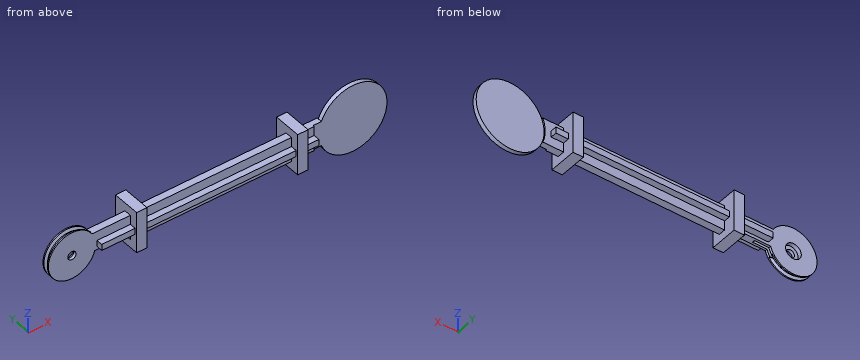
```python
from build123d import *

# Parameters (mm, degrees)
SKETCH1_R                      = 5
BOSS_EXTRUDE1_DEPTH            = 1.7
EP_CABLESLOT_DEPTH             = 0.6
SKETCH4_R                      = 1.9
EP_BALLBEARINGSLOT_DEPTH       = 1
SKETCH5_R                      = 1
EP_SHAFTHOLE_DEPTH             = 0.7
BOSS_EXTRUDE2_START            = -0.85
BOSS_EXTRUDE2_DEPTH            = 1.7
HUMERUSCLEARANCECUT_DEPTH      = 1.7
CABLECLEARANCECUT_DEPTH        = 0.6
SKETCH6_3_R                    = 8.2
MAINPLATE_DEPTH                = 0.5
FINGERPULLEYCLEARANCECUT_DEPTH = 0.35
SKETCH10_W                     = 2.5
SKETCH10_H                     = 10
BLOCK1_DEPTH                   = 3
BLOCK1_DEPTH_BACK              = 3.7
SKETCH13_W                     = 2.5
SKETCH13_H                     = 10
BLOCK2_DEPTH                   = 3
BLOCK2_DEPTH_BACK              = 3.7
SKETCH14_W                     = 36.371319344
SKETCH14_H                     = 1.5
SKETCH14_W_2                   = 5.5
STIFFENERRIB_DEPTH             = 1.5
STIFFENERRIB_DEPTH_BACK        = 3.2


with BuildPart() as part:
    # Sketch1 → Boss-Extrude1 (new body)
    with BuildSketch(Plane(origin=(0, 0, 0), x_dir=(1, 0, 0), z_dir=(0, 1, 0))):
        Circle(SKETCH1_R)
    extrude(amount=BOSS_EXTRUDE1_DEPTH)

    # Sketch2 → Revolve1 (revolve)
    with BuildSketch(Plane.XY):
        Polygon((5, 1.7), (5, 1.15), (5.7, 1.4), (5.7, 1.7), align=None)
        Polygon((5, 0.55), (5, 0), (5.7, 0), (5.7, 0.3), align=None)
    revolve(axis=Axis((0, 1.7, 0), (0, -1, 0)))

    # Sketch3 → EP_CableSlot (cut)
    with BuildSketch(Plane(origin=(0, 0.55, 0), x_dir=(1, 0, 0), z_dir=(0, 1, 0))):
        with BuildLine():
            ThreePointArc((1.166666667, -4.861984049), (2.300738274, -4.439212024), (3.3, -3.756327994))
            Line((3.3, -3.756327994), (3.3, 3.756327994))
            ThreePointArc((3.3, 3.756327994), (2.300738274, 4.439212024), (1.166666667, 4.861984049))
            ThreePointArc((1.166666667, 4.861984049), (2.270562532, 4.155468804), (2.7, 2.917190429))
            Line((2.7, 2.917190429), (2.7, -2.917190429))
            ThreePointArc((2.7, -2.917190429), (2.270562532, -4.155468804), (1.166666667, -4.861984049))
        make_face()
    extrude(amount=EP_CABLESLOT_DEPTH, mode=Mode.SUBTRACT)

    # Sketch4 → EP_BallBearingSlot (cut)
    with BuildSketch(Plane(origin=(0, 1.7, 0), x_dir=(1, 0, 0), z_dir=(0, 1, 0))):
        Circle(SKETCH4_R)
    extrude(amount=-EP_BALLBEARINGSLOT_DEPTH, mode=Mode.SUBTRACT)

    # Sketch5 → EP_ShaftHole (cut)
    with BuildSketch(Plane(origin=(0, 0.7, 0), x_dir=(1, 0, 0), z_dir=(0, 1, 0))):
        Circle(SKETCH5_R)
    extrude(amount=-EP_SHAFTHOLE_DEPTH, mode=Mode.SUBTRACT)

    # Sketch6 → Boss-Extrude2 (add)
    with BuildSketch(Plane(origin=(0, 0.85, 0), x_dir=(1, 0, 0), z_dir=(0, 1, 0)).offset(BOSS_EXTRUDE2_START)):
        with BuildLine():
            ThreePointArc((4, 3), (5, 0), (4, -3))
            Line((4, -3), (60.468486389, -3))
            ThreePointArc((60.468486389, -3), (59.9, 0), (60.468486389, 3))
            Line((60.468486389, 3), (4, 3))
        make_face()
    extrude(amount=BOSS_EXTRUDE2_DEPTH)

    # Sketch8 → HumerusClearanceCut (cut)
    with BuildSketch(Plane(origin=(0, 1.7, 0), x_dir=(1, 0, 0), z_dir=(0, 1, 0))):
        with BuildLine():
            ThreePointArc((4.846648326, 3), (5.22695702, 2.273525963), (5.499090834, 1.5))
            Line((5.499090834, 1.5), (11.499090834, 1.5))
            ThreePointArc((11.499090834, 1.5), (12.999090834, 1.901923789), (14.097167045, 3))
            Line((14.097167045, 3), (4.846648326, 3))
        make_face()
    extrude(amount=-HUMERUSCLEARANCECUT_DEPTH, mode=Mode.SUBTRACT)

    # Sketch11 → CableClearanceCut (cut)
    with BuildSketch(Plane(origin=(0, 0.55, 0), x_dir=(1, 0, 0), z_dir=(0, 1, 0))):
        with BuildLine():
            Line((8.999090834, 1.5), (5.499090834, 1.5))
            ThreePointArc((5.499090834, 1.5), (5.641017612, -0.817875483), (4.846648326, -3))
            ThreePointArc((4.846648326, -3), (4.563342119, -3.415539299), (4.2445102, -3.804488555))
            Line((4.2445102, -3.804488555), (8.999090834, 1.5))
        make_face()
        with BuildLine():
            ThreePointArc((4.846648326, -3), (5.641017612, -0.817875483), (5.499090834, 1.5))
            ThreePointArc((5.499090834, 1.5), (5.22695702, 2.273525963), (4.846648326, 3))
            Line((4.846648326, 3), (4, 3))
            ThreePointArc((4, 3), (5, 0), (4, -3))
            Line((4, -3), (4.846648326, -3))
        make_face()
    extrude(amount=CABLECLEARANCECUT_DEPTH, mode=Mode.SUBTRACT)

    # Sketch6<3> → MainPlate (add, symmetric)
    with BuildSketch(Plane(origin=(0, 0.85, 0), x_dir=(1, 0, 0), z_dir=(0, 1, 0))):
        with Locations((68.1, 0)):
            Circle(SKETCH6_3_R)
    extrude(amount=MAINPLATE_DEPTH, both=True)

    # Sketch12 → FingerPulleyClearanceCut (cut)
    with BuildSketch(Plane(origin=(0, 0, 0), x_dir=(1, 0, 0), z_dir=(0, 1, 0))):
        with BuildLine():
            ThreePointArc((60.468486389, -3), (59.9, 0), (60.468486389, 3))
            Line((60.468486389, 3), (58.468486389, 3))
            Line((58.468486389, 3), (58.468486389, -3))
            Line((58.468486389, -3), (60.468486389, -3))
        make_face()
    extrude(amount=FINGERPULLEYCLEARANCECUT_DEPTH, mode=Mode.SUBTRACT)

    # Sketch10 → Block1 (add, two sides)
    with BuildSketch(Plane(origin=(0, 1.7, 0), x_dir=(1, 0, 0), z_dir=(0, 1, 0))) as block1_sk:
        with Locations((15.347167045, 0)):
            Rectangle(SKETCH10_W, SKETCH10_H)
    extrude(amount=BLOCK1_DEPTH)
    extrude(block1_sk.sketch, amount=-BLOCK1_DEPTH_BACK)

    # Sketch13 → Block2 (add, two sides)
    with BuildSketch(Plane(origin=(0, 1.7, 0), x_dir=(1, 0, 0), z_dir=(0, 1, 0))) as block2_sk:
        with Locations((54.218486389, 0)):
            Rectangle(SKETCH13_W, SKETCH13_H)
    extrude(amount=BLOCK2_DEPTH)
    extrude(block2_sk.sketch, amount=-BLOCK2_DEPTH_BACK)

    # Sketch14 → StiffenerRib (add, two sides)
    with BuildSketch(Plane(origin=(0, 1.7, 0), x_dir=(1, 0, 0), z_dir=(0, 1, 0))) as stiffenerrib_sk:
        with BuildLine():
            Line((16.597167045, -0.75), (16.597167045, 0.75))
            Line((16.597167045, 0.75), (6.053717866, 0.75))
            ThreePointArc((6.053717866, 0.75), (6.1, 0), (6.053717866, -0.75))
            Line((6.053717866, -0.75), (16.597167045, -0.75))
        make_face()
        with Locations((34.782826717, 0)):
            Rectangle(SKETCH14_W, SKETCH14_H)
        with Locations((55.718486389, 0)):
            Rectangle(SKETCH14_W_2, SKETCH14_H)
    extrude(amount=STIFFENERRIB_DEPTH)
    extrude(stiffenerrib_sk.sketch, amount=-STIFFENERRIB_DEPTH_BACK)


solid = part.part
```
CAD build for the part. Positions are in the model's coordinates, mm. Give positions to 0.01 mm unless a question says otherwise; leave off trailing zeros. Write each loop counter-clockwise with the first axis right and the second up, starting at its lowest first coordinate (ties: lowest second). Pieces come first, ordered by that corner, then holes. Notation, with made-up numbers: M -14.75,-14.5 L -2.75,-14.5 A32 ccw -2.75,18.5 Z; hole C -8.75,-21.75 d2. An arc over 180 degrees is marked long. Return JSON: item names as keys, results as strings. Group by question number.
(1) Band-saw the part on D-D (x = 68.1). Give the cut face in (y, z).
(2) Band-saw the part on B-B (x = 25). Give the cut face in (y, z), and give its area (3 significant figures).
(3) Band-saw the part on C-C (z = 0). State how many separate pieces and enclosed holes the cut face has, and give its area (3 significant figures).
(4) Band-saw the part on A-A (x = 0). Give the cut face in (y, z).
(5) Flat gauge pins, fed straight in: pin 1 Ø1.5 at (x, z) = (5.5, -0.5) entering from -Y; pin 2 Ø1.2 at (x, y) = (38, 2.5) entering from +Z; pin 3 Ø1.2 at (x, y) = (9.5, -1) entering from -Z. Where does each tip first touch, or does it go through?
(6) Drill centre lines: L1, parallel to X at y = 1, z = 0; L2, parallel to X at y = 2.25, z = -2.25; L3, parallel to Z at x = 0, y = 0.2. Where is each one in solid material? Low to high. Write a range as [from, to].
Entries:
{
 "1": {"outline": "M 0.35,-8.2 L 1.35,-8.2 L 1.35,8.2 L 0.35,8.2 Z"},
 "2": {"outline": "M -1.5,-0.75 L 0,-0.75 L 0,-3 L 1.7,-3 L 1.7,-0.75 L 3.2,-0.75 L 3.2,0.75 L 1.7,0.75 L 1.7,3 L 0,3 L 0,0.75 L -1.5,0.75 Z", "area": "14.7 mm^2"},
 "3": {"separate pieces": "2", "enclosed holes": "2", "area": "288 mm^2"},
 "4": {"outline": "M 0,-5.7 L 0.3,-5.7 L 0.55,-5 L 1.15,-5 L 1.4,-5.7 L 1.7,-5.7 L 1.7,-1.9 L 0.7,-1.9 L 0.7,-1 L 0,-1 Z; M 0,1 L 0.7,1 L 0.7,1.9 L 1.7,1.9 L 1.7,5.7 L 1.4,5.7 L 1.15,5 L 0.55,5 L 0.3,5.7 L 0,5.7 Z"},
 "5": {"pin 1": "stops at y = -1.5", "pin 2": "stops at z = 0.75", "pin 3": "stops at z = -0.75"},
 "6": {"L1": "x = [-5, -1.9], [1.9, 2.7], [3.3, 5], [6.1, 76.3]", "L2": "x = [14.1, 16.6], [52.97, 55.47]", "L3": "z = [-5.7, -1], [1, 5.7]"}
}
